Can you work these out from the model? Positions are in its coordinate system, mm. A direction names the side the tool comes from. Coordinates: 2 decimals unless noted, no trailing zeros. Order: outer loops, then holes, each group sorted by start corner. A loop starts at its lowest first (then second) coordinate and runs counter-clockwise, first axis right, second up. Notation, with made-up numbers: (63, -21.5) -> (105, -21.5) arc R35 ccw to (105, 16.5) -> close; hole circle Ø4 at (59, 42.5). An arc over 180 degrees is marked (long way). Use a Markdown table: item, result. Add a question column.
1. Suppose I cut it at A-A, the plane x = 0. List the corners of the cut face in (y, z) for me.
2. Suppose I cut it at D-D, the plane y = -11.5. List the corners of the cut face in (x, z) for me, then the cut area to 3 significant figures.
3. For faces 4 (the flat face through (1.941, 11, 10)), 5 (the flat face through (0, 0, 18.8)), which set-ups out of +Z, -Z, +X, -X, +Y, -Y let a thin tool reach every point of the face, with its end or its side?
4. Suppose I cut it at C-C, the plane y = 1. List the corners of the cut face in (x, z) for me.
5. We'd pull the mould along X, two halves only. Please class faces 1 (the flat face through (0, 0, 0.8)), 2 (the cylindrical face through (-5.35, -24.08, 9.67)), 3 (the flat face through (-3, -10.127, 10)): pulls with the +X half, pulls with the -X half, needs draft (parallel to the pull), parting line crosses it, or undercut.
6. If I drill on line 1 along Y through (x, z) = (-2.5, 15.5); line 2 along X through (y, z) = (2, 5.75); line 3 along Y through (x, z) = (1, 14), over which ranges is the centre line in solid material (lowest first)? Write a range as from..to.
7. Suppose I cut it at B-B, the plane z = 2. List the corners of the cut face in (x, y) for me.
8. For pin 1 Ø3 at (x, z) = (10.5, 9.5) entering from -Y; pin 2 Ø5 at (x, z) = (-3, 6) entering from -Y; pin 3 Ø1.5 at (x, z) = (-2.5, 12) entering from +Y, each with a flat end and sliding along its axis, tell me the tip position at first contact or that it passes through.
```python
from build123d import *

# Parameters (mm, degrees)
F0_R     = 24.66759
F0_W     = 9.8689098377
F0_H     = 3.4395875409
F0_W_2   = 9.86891
F0_H_2   = 3.43959
F1_DEPTH = 18.8
F2_DEPTH = 0.8


# Not quite as in the source:
# - a feature names something its author has since deleted; it is built from what else it names


with BuildPart() as f1:
    # F0 (on Top) → F1 (new body)
    with BuildSketch(Plane.XY):
        Circle(F0_R)
        with Locations((-2.9931267491, -8.4071261808)):
            Rectangle(F0_W, F0_H, mode=Mode.SUBTRACT)
        with Locations((-8.8684857703, 1.2023462914)):
            Rectangle(F0_W_2, F0_H_2, mode=Mode.SUBTRACT)
        with Locations((-2.9931267491, 10.8118187636)):
            Rectangle(F0_W, F0_H, mode=Mode.SUBTRACT)
        with BuildLine():
            Line((11.3292662427, 3.3551587258), (11.3292662427, -0.9376045782))
            Line((11.3292662427, -0.9376045782), (7.332555484, -0.9376045782))
            ThreePointArc((7.332555484, -0.9376045782), (5.186173832, 1.2087770738), (7.332555484, 3.3551587258))
            Line((7.332555484, 3.3551587258), (11.3292662427, 3.3551587258))
        make_face(mode=Mode.SUBTRACT)
    extrude(amount=F1_DEPTH)

    # F0 (on Top) → F2 (cut)
    with BuildSketch(Plane.XY):
        Circle(F0_R)
        with Locations((-2.9931267491, -8.4071261808)):
            Rectangle(F0_W, F0_H, mode=Mode.SUBTRACT)
        with Locations((-8.8684857703, 1.2023462914)):
            Rectangle(F0_W_2, F0_H_2, mode=Mode.SUBTRACT)
        with Locations((-2.9931267491, 10.8118187636)):
            Rectangle(F0_W, F0_H, mode=Mode.SUBTRACT)
        with BuildLine():
            Line((11.3292662427, 3.3551587258), (11.3292662427, -0.9376045782))
            Line((11.3292662427, -0.9376045782), (7.332555484, -0.9376045782))
            ThreePointArc((7.332555484, -0.9376045782), (5.186173832, 1.2087770738), (7.332555484, 3.3551587258))
            Line((7.332555484, 3.3551587258), (11.3292662427, 3.3551587258))
        make_face(mode=Mode.SUBTRACT)
        with Locations((-2.9931267491, -8.4071261808)):
            Rectangle(F0_W, F0_H)
    extrude(amount=F2_DEPTH, mode=Mode.SUBTRACT)


solid = f1.part
```
Worked out:
| question | item | result |
|---|---|---|
| 1 | outline | (-24.67, 0.8) -> (-10.13, 0.8) -> (-10.13, 18.8) -> (-24.67, 18.8) -> close; (-6.69, 0.8) -> (9.09, 0.8) -> (9.09, 18.8) -> (-6.69, 18.8) -> close; (12.53, 0.8) -> (24.67, 0.8) -> (24.67, 18.8) -> (12.53, 18.8) -> close |
| 2 | outline | (-21.82, 0.8) -> (21.82, 0.8) -> (21.82, 18.8) -> (-21.82, 18.8) -> close |
| 2 | area | 786 mm² |
| 3 | face 4 | +Z, -Z |
| 3 | face 5 | +Z, +X, -X, +Y, -Y |
| 4 | outline | (-24.65, 0.8) -> (-13.8, 0.8) -> (-13.8, 18.8) -> (-24.65, 18.8) -> close; (-3.93, 0.8) -> (5.2, 0.8) -> (5.2, 18.8) -> (-3.93, 18.8) -> close; (11.33, 0.8) -> (24.65, 0.8) -> (24.65, 18.8) -> (11.33, 18.8) -> close |
| 5 | face 1 | needs draft |
| 5 | face 2 | parting line crosses it |
| 5 | face 3 | undercut |
| 6 | line 1 | y = -24.54..-10.13, -6.69..9.09, 12.53..24.54 |
| 6 | line 2 | x = -24.59..-13.8, -3.93..5.34, 11.33..24.59 |
| 6 | line 3 | y = -24.65..-10.13, -6.69..9.09, 12.53..24.65 |
| 7 | outline | circle Ø49.34 at (0, 0); hole (-13.8, -0.52) -> (-3.93, -0.52) -> (-3.93, 2.92) -> (-13.8, 2.92) -> close; hole (-7.93, -10.13) -> (1.94, -10.13) -> (1.94, -6.69) -> (-7.93, -6.69) -> close; hole (-7.93, 9.09) -> (1.94, 9.09) -> (1.94, 12.53) -> (-7.93, 12.53) -> close; hole (7.33, -0.94) -> (11.33, -0.94) -> (11.33, 3.36) -> (7.33, 3.36) arc R2.15 ccw to start |
| 8 | pin 1 | stops at y = -22.97 |
| 8 | pin 2 | stops at y = -24.66 |
| 8 | pin 3 | stops at y = 24.61 |
